For this review, take the finished solid that the model builds, in its own axes (mm). Give positions to 0.01 mm unless a question says otherwise; leave off trailing zeros. Order: outer loops, then holes, each group sorted by start corner. A loop starts at its lowest first (then second) coordinate and runs counter-clockwise, first axis right, second up. Notation, with made-up numbers: (13, -26.5) - (57, -26.5) arc R28 ccw to (57, 0.5) - close; hole circle Ø1 at (3, 89). An arc over 180 degrees is marked (long way). One line per item, written item: value.
```python
from build123d import *

# Parameters (mm, degrees)
SKETCH_1_W      = 450
SKETCH_1_H      = 750
SKETCH_1_W_2    = 20
SKETCH_1_H_2    = 650
EXTRUDE_1_DEPTH = 10


with BuildPart() as part:
    # Эскиз1 → Бобышка-Вытянуть1 (new body)
    with BuildSketch(Plane(origin=(0, 0, 0), x_dir=(1, 0, 0), z_dir=(0, 1, 0))):
        Rectangle(SKETCH_1_W, SKETCH_1_H)
        with Locations((0, -25)):
            Rectangle(SKETCH_1_W_2, SKETCH_1_H_2, mode=Mode.SUBTRACT)
    extrude(amount=EXTRUDE_1_DEPTH)


solid = part.part
```
(1) Wall thickness on line 1 (X direction, y = 3, z = -7): over which ranges is the line inside the solid? List them lowest first. Write a range as from..to.
Answers below:
line 1: x = -225..-10, 10..225
(2) Take a section at A-A (z = -56). Write out the cut boundary in (x, y).
Answers below:
outline: (-225, 0) - (-10, 0) - (-10, 10) - (-225, 10) - close; (10, 0) - (225, 0) - (225, 10) - (10, 10) - close
(3) Take a section at B-B (x = 1). Write out the cut boundary in (y, z), then the cut area to 3 significant figures.
Answers below:
outline: (0, -375) - (10, -375) - (10, -300) - (0, -300) - close; (0, 350) - (10, 350) - (10, 375) - (0, 375) - close
area: 1,000 mm^2
(4) Take a section at C-C (y = 5). Write out the cut boundary in (x, z).
Answers below:
outline: (-225, -375) - (225, -375) - (225, 375) - (-225, 375) - close; hole (-10, -300) - (10, -300) - (10, 350) - (-10, 350) - close
(5) Draft analysis for pull direction Y (two halves, no side actions). For faces 1 (the face through (47, 0, -5)), 2 (the face through (47, 10, -5)), state which applies: pulls with the +Y half, pulls with the -Y half, needs draft (parallel to the pull), parting line crosses it, or undercut.
Answers below:
face 1: pulls with the -Y half
face 2: pulls with the +Y half
